For this review, take the finished solid that the model builds, in its own axes (mm). A direction names the side the tool comes from. Coordinates: 2 decimals unless noted, no trailing zeros. Write each loop counter-clockwise with the first axis right and the second up, starting at its lowest first coordinate (ties: lowest second). Pieces come first, ordered by that corner, then holes. Notation, with made-up numbers: M -0.5,4.5 L 12.5,4.5 A29 ccw 12.5,42.5 Z; hole C 1.5,38.25 d11. An arc over 180 degrees is marked long. One line per question, with ' | ' between items.
from build123d import *

# Parameters (mm, degrees)
EXTRUDE_1_DEPTH     = 4
EXTRUDE_2_DEPTH     = 5
CUT_EXTRUDE_1_DEPTH = 5
CUT_EXTRUDE_3_DEPTH = 5
EXTRUDE_3_DEPTH     = 4
SKETCH_8_W          = 12
SKETCH_8_H          = 4
CUT_EXTRUDE_4_DEPTH = 1
SKETCH_9_R          = 1.4
CUT_EXTRUDE_5_DEPTH = 4


with BuildPart() as part:
    # 草图1 → 凸台-拉伸1 (new body)
    with BuildSketch(Plane.XY):
        Polygon((-15.155444566, 17.5), (15.155444566, -35), (15.155444566, 35), align=None)
    extrude(amount=EXTRUDE_1_DEPTH)

    # 草图3 → 凸台-拉伸2 (add)
    with BuildSketch(Plane(origin=(-11.366583425, 19.6875, 0), x_dir=(0.8660254037844398, 0.499999999999998, 0), z_dir=(-0.49999999999999806, 0.8660254037844399, 0))):
        Polygon((7.125, -4), (13.125, -4), (19.125, -4), (19.125, 0), (7.125, 0), align=None)
    extrude(amount=EXTRUDE_2_DEPTH)

    # 草图4 → 切除-拉伸1 (cut)
    with BuildSketch(Plane(origin=(117.013646285, -126.133628904, 5), x_dir=(0.9999710727819138, 0.007606155361845417, 0), z_dir=(0, 0, 1))):
        Polygon((-106.588705014, 124.032873802), (-111.52268914, 132.7309081), (-115.871706289, 130.263916037), (-110.937722163, 121.565881739), align=None)
    extrude(amount=-CUT_EXTRUDE_1_DEPTH, mode=Mode.SUBTRACT)

    # 草图6 → 切除-拉伸3 (cut)
    with BuildSketch(Plane(origin=(116.750820958, -91.580334705, 5), x_dir=(0.9999710727819138, 0.007606155361845417, 0), z_dir=(0, 0, 1))):
        Polygon((-113.442317429, 112.033605516), (-110.481926953, 106.814784937), (-106.132909805, 109.281777), (-109.09330028, 114.500597579), align=None)
    extrude(amount=-CUT_EXTRUDE_3_DEPTH, mode=Mode.SUBTRACT)

    # 草图7 → 凸台-拉伸3 (add)
    with BuildSketch(Plane(origin=(0, 0, 0), x_dir=(-1, 0, 0), z_dir=(0, 0, -1))):
        Polygon((15.155444566, 17.5), (-15.155444566, -35), (-8.084376754, -42.071067812), align=None)
    extrude(amount=-EXTRUDE_3_DEPTH)

    # 草图8 → 切除-拉伸4 (cut)
    with BuildSketch(Plane(origin=(-13.866583425, 24.017627019, 0), x_dir=(0.8660254037844398, 0.49999999999999806, 0), z_dir=(-0.499999999999998, 0.8660254037844397, 0))):
        with Locations((13.125, -2)):
            Rectangle(SKETCH_8_W, SKETCH_8_H)
    extrude(amount=-CUT_EXTRUDE_4_DEPTH, mode=Mode.SUBTRACT)

    # 草图9 → 切除-拉伸5 (cut)
    with BuildSketch(Plane(origin=(116.744731615, -90.779776973, 0), x_dir=(-0.9999710727819138, -0.007606155361845545, 0), z_dir=(0, 0, -1))):
        with Locations(Location((117.644385016, 103.100964858, 0), (0, 0, 0.435804803))):
            Circle(SKETCH_9_R)
    extrude(amount=-CUT_EXTRUDE_5_DEPTH, mode=Mode.SUBTRACT)


solid = part.part
1. For line 1 along Y through (x, z) = (8.5, 1.65); line 2 along X through (y, z) = (10.5, 1.9); line 3 along X through (y, z) = (16.5, 3.75), list the stretches that pass through material, from the lowest coordinate up.
Computed values:
line 1: y = -41.66 to -3.48, -1.21 to 16.15, 19.12 to 31.16 | line 2: x = -12.42 to -2.73, -0.63 to 15.16 | line 3: x = -14.77 to 4.24, 9.11 to 15.16
2. Take a section at B-B on x = -1.5. State the section outline as (y, z) points, plus the area to 3 significant figures.
Computed values:
outline: M -17.5,0 L 10.04,0 L 10.04,4 L -17.5,4 Z; M 12.81,0 L 30,0 L 30,4 L 12.81,4 Z | area: 179 mm2
3. Take a section at A-A on z = 1.3. State the section outline as (x, y) points.
Computed values:
outline: M -15.16,17.5 L 8.08,-42.07 L 15.16,-35 L 15.16,35 L 5.2,29.25 L 3.2,32.71 L -7.2,26.71 L -5.2,23.25 Z; hole C -1.68,11.42 d2.8; hole M 0.15,3.25 L 5.15,-5.42 L 9.48,-2.92 L 4.48,5.75 Z; hole M 2.46,19.59 L 5.46,14.39 L 9.79,16.89 L 6.79,22.09 Z
4. Take a section at D-D on x = 11. State the section outline as (y, z) points.
Computed values:
outline: M -39.16,0 L 32.6,0 L 32.6,4 L -39.16,4 Z
5. Machinability: for faces 1 (the flat face through (11.669, -38.486, 1.972)), 2 (the flat face through (4.21, 30.96, 2.03)), 3 (the flat face through (-10.106, 20.415, 1.972)), 4 (the flat face through (3.939, 17.025, 2.028)), which of the approach directions +Z, -Z, +X, -X, +Y, -Y give a long, thin tool a straight path to every point of the face, cutting with its end or side? Answer none if there is none.
Computed values:
face 1: +Z, -Z, +X, -Y | face 2: +Z, -Z, +Y | face 3: +Z, -Z, -X | face 4: +Z, -Z
6. Take a section at C-C on y = -11. State the section outline as (x, z) points, plus the area to 3 significant figures.
Computed values:
outline: M -4.04,0 L 15.16,0 L 15.16,4 L -4.04,4 Z | area: 76.8 mm2
7. Clearance check with a flat-ended pin moving along its axis: P1, Ø1.5, axis at x = -6.5, z = 1, coming from the +Y side. State where the tip first meets the part, or that it passes through.
Computed values:
P1: stops at y = 27.55
